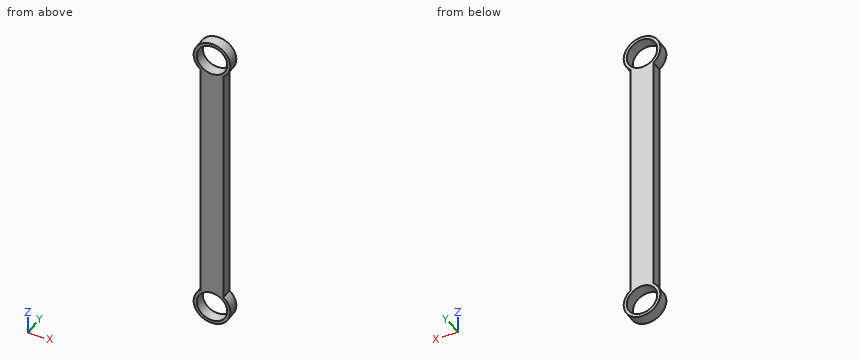
from build123d import *

# Parameters (mm, degrees)
F0_R     = 4.2291
F1_DEPTH = 3.175


with BuildPart() as f1:
    # F0 (on Front) → F1 (new body)
    with BuildSketch(Plane.XZ):
        with BuildLine():
            ThreePointArc((-3.175, -34.134426), (0, -33.02), (3.175, -34.134426))
            Line((3.175, -34.134426), (3.175, 0))
            Line((3.175, 0), (-3.175, 0))
            Line((-3.175, 0), (-3.175, -34.134426))
        make_face()
        with BuildLine():
            ThreePointArc((5.08, -38.1), (4.57905, -35.900295), (3.175, -34.134426))
            ThreePointArc((3.175, -34.134426), (0, -33.02), (-3.175, -34.134426))
            ThreePointArc((-3.175, -34.134426), (-2.199705, -42.67905), (5.08, -38.1))
        make_face()
        with Locations((0, -38.1)):
            Circle(F0_R, mode=Mode.SUBTRACT)
        with BuildLine():
            Line((-3.175, 0), (3.175, 0))
            Line((3.175, 0), (3.175, 34.134426))
            ThreePointArc((3.175, 34.134426), (0, 33.02), (-3.175, 34.134426))
            Line((-3.175, 34.134426), (-3.175, 0))
        make_face()
        with BuildLine():
            ThreePointArc((-3.175, 34.134426), (0, 33.02), (3.175, 34.134426))
            ThreePointArc((3.175, 34.134426), (4.57905, 35.900295), (5.08, 38.1))
            ThreePointArc((5.08, 38.1), (-2.199705, 42.67905), (-3.175, 34.134426))
        make_face()
        with Locations((0, 38.1)):
            Circle(F0_R, mode=Mode.SUBTRACT)
    extrude(amount=F1_DEPTH)


solid = f1.part
Read the model definition and answer for the solid it produces. Units are mm, in the model's axes. Give positions to 0.01 mm unless a question says otherwise; leave off trailing zeros. Write each loop counter-clockwise with the first axis right and the second up, starting at its lowest first coordinate (ties: lowest second). Pieces come first, ordered by that corner, then holes. Notation, with made-up numbers: (81.25, 73.25) - (103.25, 73.25) arc R18 ccw to (103.25, 77.25) - close; hole circle Ø3 at (43, 23). An arc over 180 degrees is marked (long way). Use CSV: the item, a comma, the result in double quotes. Start each with the question number.
(1) Find section C-C (z = 25). Give the vertices of the cut face in (x, y) (3 decimals).
(2) Find section B-B (y = -2.4). Give the vertices of the cut face in (x, z) (3 decimals), plus the area to 3 significant figures.
(3) Given P1, Ø1, axis at x = 1, y = -1.5, coming from the -Z side; P2, Ø1, axis at y = -1.5, z = -34, coming from the -X side; P3, Ø5, axis at x = 0, z = -38.1, coming from the +Y side, each flat-ended and moving along its own axis, determine where each tip first touches the part or whether it passes through.
(4) Find section A-A (x = 0). Give the vertices of the cut face in (y, z) (3 decimals), plus the area to 3 significant figures.
(5) Consider line 1 along Z through (x, y) = (0, -1.05); line 2 along Z through (x, y) = (2.75, -2.2); line 3 along X through (y, z) = (-1.4, -18.5) (3 decimals). Determine where each line is inside the solid, lowest interval first.
Findings below:
1,outline,"(-3.175, -3.175) - (3.175, -3.175) - (3.175, 0) - (-3.175, 0) - close"
2,outline,"(-3.175, -34.134) arc R5.08 ccw (long way) to (3.175, -34.134) - (3.175, 34.134) arc R5.08 ccw (long way) to (-3.175, 34.134) - close; hole circle Ø8.458 at (0, -38.1); hole circle Ø8.458 at (0, 38.1)"
2,area,"474 mm2"
3,P1,"z = -43.16"
3,P2,"x = -3.58"
3,P3,"through"
4,outline,"(-3.175, -43.18) - (0, -43.18) - (0, -42.329) - (-3.175, -42.329) - close; (-3.175, -33.871) - (0, -33.871) - (0, 33.871) - (-3.175, 33.871) - close; (-3.175, 42.329) - (0, 42.329) - (0, 43.18) - (-3.175, 43.18) - close"
4,area,"220 mm2"
5,line 1,"-43.18 to -42.33, -33.87 to 33.87, 42.33 to 43.18"
5,line 2,"-42.37 to -41.31, -34.89 to 34.89, 41.31 to 42.37"
5,line 3,"-3.175 to 3.175"
